from build123d import *

# Parameters (mm, degrees)
SKETCH1_W           = 33.02
SKETCH1_H           = 25.4
BOSS_EXTRUDE1_DEPTH = 25.4
CUT_EXTRUDE2_START  = -3.81
SKETCH1_4_W         = 15.875
SKETCH1_4_H         = 0.508
SKETCH1_4_W_2       = 27.94
SKETCH1_4_H_2       = 5.08
CUT_EXTRUDE2_DEPTH  = 2.54
SKETCH1_3_W         = 27.94
SKETCH1_3_H         = 13.97
CUT_EXTRUDE1_DEPTH  = 6.35
CUT_EXTRUDE3_START  = -6.35
SKETCH1_5_W         = 15.875
SKETCH1_5_H         = 2.667
SKETCH1_5_H_2       = 0.508
CUT_EXTRUDE3_DEPTH  = 19.05
SKETCH4_W           = 12.7
SKETCH4_H           = 3.175
CUT_EXTRUDE4_DEPTH  = 19.05
CUT_EXTRUDE5_DEPTH  = 6.35


with BuildPart() as part:
    # Sketch1 → Boss-Extrude1 (new body)
    with BuildSketch(Plane.XY):
        with Locations((-2.974473684, 2.395175439)):
            Rectangle(SKETCH1_W, SKETCH1_H)
    extrude(amount=-BOSS_EXTRUDE1_DEPTH)

    # Sketch1_4 → Cut-Extrude2 (cut)
    with BuildSketch(Plane.XY.offset(CUT_EXTRUDE2_START)):
        Polygon((-10.911973684, -6.494824561), (-16.944473684, -6.494824561), (-16.944473684, -7.764824561), (10.995526316, -7.764824561), (10.995526316, -6.494824561), (4.963026316, -6.494824561), (4.963026316, -7.002824561), (-10.911973684, -7.002824561), align=None)
        with Locations((-2.974473684, -6.748824561)):
            Rectangle(SKETCH1_4_W, SKETCH1_4_H)
        with Locations((-2.974473684, 10.015175439)):
            Rectangle(SKETCH1_4_W_2, SKETCH1_4_H_2)
    extrude(amount=-CUT_EXTRUDE2_DEPTH, mode=Mode.SUBTRACT)

    # Sketch1_3 → Cut-Extrude1 (cut)
    with BuildSketch(Plane.XY):
        with Locations((-2.974473684, 0.490175439)):
            Rectangle(SKETCH1_3_W, SKETCH1_3_H)
    extrude(amount=-CUT_EXTRUDE1_DEPTH, mode=Mode.SUBTRACT)

    # Sketch1_5 → Cut-Extrude3 (cut)
    with BuildSketch(Plane.XY.offset(CUT_EXTRUDE3_START)):
        with Locations((-2.974473684, -5.161324561)):
            Rectangle(SKETCH1_5_W, SKETCH1_5_H)
        with Locations((-2.974473684, -6.748824561)):
            Rectangle(SKETCH1_5_W, SKETCH1_5_H_2)
    extrude(amount=-CUT_EXTRUDE3_DEPTH, mode=Mode.SUBTRACT)

    # Sketch4 → Cut-Extrude4 (cut)
    with BuildSketch(Plane(origin=(-10.911973684, 0, 0), x_dir=(0, 0, -1), z_dir=(1, 0, 0))):
        with Locations((12.7, -5.415324561)):
            Rectangle(SKETCH4_W, SKETCH4_H)
    extrude(amount=-CUT_EXTRUDE4_DEPTH, mode=Mode.SUBTRACT)

    # Sketch7 → Cut-Extrude5 (cut)
    with BuildSketch(Plane(origin=(-16.944473684, 0, 0), x_dir=(0, 0, -1), z_dir=(1, 0, 0))):
        Polygon((0, 7.475175439), (3.81, 7.475175439), (3.81, 12.555175439), (6.35, 12.555175439), (6.35, -7.764824561), (3.81, -7.764824561), (3.81, -6.494824561), (0, -6.494824561), align=None)
    extrude(amount=-CUT_EXTRUDE5_DEPTH, mode=Mode.SUBTRACT)


solid = part.part
Model file for the job. Use its own axes, mm. A direction names the side the tool comes from. Coordinates: 2 decimals unless noted, no trailing zeros. Write each loop counter-clockwise with the first axis right and the second up, starting at its lowest first coordinate (ties: lowest second). Pieces come first, ordered by that corner, then holes. Notation, with made-up numbers: (89, -32) -> (131, -32) arc R13 cw to (131, -17) -> close; hole circle Ø9 at (-21, 84). An arc over 180 degrees is marked (long way). One line per item, written item: value. Start each with the question number.
1) Pull direction Z, two halves, no side cores. Call faces 4 (the face through (-3, 3, -25.4)), 5 (the face through (-4, -6.495, -2)), 6 (the face through (-4, -7, -3.81)): +Z half, -Z half, draft (parallel to the pull), parting line (faces both ways), or undercut.
2) Slice it at D-D on x = 9. Write the cut outline in (y, z), then the cut area to 3 significant figures.
3) Flat gauge pin, fed straight in: pin 1 Ø10 at (x, y) = (-4.5, 1.5) entering from +Z. Where does the tip first touch, or does it go through?
4) Which spindle directions (+Z, -Z, +X, -X, +Y, -Y) get a long thin tool onto all of the face, cutting with end or side? Do faces 1 (the face through (-7, -3.828, -16)), 2 (the face through (-15, -5, -19.05)), 3 (the face through (-4, 7.475, -2)). Say none if no direction does.
5) Probe probe 1 along Y at (x, z) = (-4, -10.75); probe 2 along Z at (x, y) = (-17, 12.5); probe 3 along Y at (x, z) = (-7, -2.25). List the from-to ranges inside material, lowest first.
6) Slice it at B-B on z = -19.5. Write the cut outline in (x, y), then the cut area to 3 significant figures.
7) Slice it at C-C on y = -6. Write the cut outline in (x, z), then the cut area to 3 significant figures.
8) Slice it at A-A on x = 2. Write the cut outline in (y, z).
Answers follow:
1. face 4: -Z half
1. face 5: draft
1. face 6: undercut
2. outline: (-10.3, -25.4) -> (15.1, -25.4) -> (15.1, 0) -> (7.48, 0) -> (7.48, -3.81) -> (12.56, -3.81) -> (12.56, -6.35) -> (-7.76, -6.35) -> (-7.76, -3.81) -> (-6.49, -3.81) -> (-6.49, 0) -> (-10.3, 0) -> close
2. area: 540 mm2
3. pin 1: z = -6.35
4. face 1: +Z
4. face 2: -X
4. face 3: +Z, -X
5. probe 1: -10.3 to -7, -3.83 to 15.1
5. probe 2: -25.4 to -6.35, -3.81 to 0
5. probe 3: -10.3 to -6.49, 7.48 to 15.1
6. outline: (-19.48, -10.3) -> (13.54, -10.3) -> (13.54, 15.1) -> (-19.48, 15.1) -> close; hole (-10.91, -7) -> (4.96, -7) -> (4.96, -3.83) -> (-10.91, -3.83) -> close
6. area: 788 mm2
7. outline: (-19.48, -25.4) -> (-10.91, -25.4) -> (-10.91, -19.05) -> (-19.48, -19.05) -> close; (4.96, -25.4) -> (13.54, -25.4) -> (13.54, 0) -> (11, 0) -> (11, -6.35) -> (4.96, -6.35) -> close
7. area: 234 mm2
8. outline: (-10.3, -25.4) -> (-7, -25.4) -> (-7, -6.35) -> (-7.76, -6.35) -> (-7.76, -3.81) -> (-6.49, -3.81) -> (-6.49, 0) -> (-10.3, 0) -> close; (-3.83, -25.4) -> (15.1, -25.4) -> (15.1, 0) -> (7.48, 0) -> (7.48, -3.81) -> (12.56, -3.81) -> (12.56, -6.35) -> (-3.83, -6.35) -> close
